Part model, mm, in its own coordinate system. A direction names the side the tool comes from. Give positions to 0.01 mm unless a question says otherwise; leave off trailing zeros. Write each loop counter-clockwise with the first axis right and the second up, starting at its lowest first coordinate (ties: lowest second). Pieces come first, ordered by that corner, then holes. Notation, with made-up numbers: M 3.25,52.25 L 21.25,52.25 A14 ccw 21.25,59.25 Z; hole C 58,84 d1. An arc over 180 degrees is marked long. Answer as CSV lines item,"result". Start each with the question number.
Item 1: Band-saw the part on C-C, the plane y = 0. Count the separate pieces of the cut face and the enclosed holes in it, then the cut area to 3 significant figures.
Item 2: Wall check: L1, parallel to Y at x = -40, z = 1.25 (3 decimals); L2, parallel to X at y = -12.5, z = 2; L3, parallel to Y at x = 14.5, z = 1.25. Give the ranges that are in metal, low to high. Write a range as from..to.
Item 3: Band-saw the part on B-B, the plane y = -10. List the corners of the cut face in (x, z).
Item 4: 3-axis set-ups, long thin cutter, end or side, ignore diameter. For faces 5 (the flat face through (0, 2.5, 19)), 6 (the cylindrical face through (-45.245, 25.361, 1.232)), 7 (the cylindrical face through (27.15, 26.99, 10.9)): which of +Z, -Z, +X, -X, +Y, -Y reach the whole face in a straight line?
Item 5: Two-plate mould, pull along X, no slides. Class faces 1 (the cylindrical face through (-25.361, -25.245, 9.895)), 2 (the cylindrical face through (46.99, -27.15, 1.73)), 3 (the cylindrical face through (-27.15, -26.99, 10.9)), 4 (the flat face through (34, 0, 5)): +X half, -X half, draft (parallel to the pull), parting line (faces both ways), or undercut.
Item 6: Pin check, flat tips, straight feed: pin 1 (10 mm diameter, centred on x = 40, y = 0, fed in from +Z); pin 2 (18.5 mm diameter, centred on x = 37, y = -9.5, fed in from +Z); pin 3 (3 mm diameter, centred on y = -10, z = 11.5, fed in from -X); pin 4 (10 mm diameter, centred on x = -38.5, y = -13.5, fed in from -Z). Stop position of each tip, or through.
Item 7: Band-saw the part on A-A, the plane z = 14.5. List the corners of the cut face in (x, y), then the cut area to 3 significant figures.
from build123d import *

# Parameters (mm, degrees)
F0_R     = 4.345
F1_DEPTH = 5
F3_DEPTH = 15
F4_T     = -2.5
F5_W     = 45
F5_H     = 5
F6_DEPTH = 20.001
F7_R     = 1.5


with BuildPart() as f1:
    # F0 (on Top) → F1 (new body)
    with BuildSketch(Plane.XY):
        with BuildLine():
            Line((40, 30), (-40, 30))
            ThreePointArc((-40, 30), (-47.0710678119, 27.0710678119), (-50, 20))
            Line((-50, 20), (-50, -20))
            ThreePointArc((-50, -20), (-47.0710678119, -27.0710678119), (-40, -30))
            Line((-40, -30), (40, -30))
            ThreePointArc((40, -30), (47.0710678119, -27.0710678119), (50, -20))
            Line((50, -20), (50, 20))
            ThreePointArc((50, 20), (47.0710678119, 27.0710678119), (40, 30))
        make_face()
        with Locations((-40, 0)):
            Circle(F0_R, mode=Mode.SUBTRACT)
        with Locations((40, 0)):
            Circle(F0_R, mode=Mode.SUBTRACT)
    extrude(amount=F1_DEPTH)

    # F2 (on face) → F3 (join)
    with BuildSketch(Plane.XY.offset(5)):
        with BuildLine():
            Line((20, 30), (-20, 30))
            ThreePointArc((-20, 30), (-27.0710678119, 27.0710678119), (-30, 20))
            Line((-30, 20), (-30, -20))
            ThreePointArc((-30, -20), (-27.0710678119, -27.0710678119), (-20, -30))
            Line((-20, -30), (20, -30))
            ThreePointArc((20, -30), (27.0710678119, -27.0710678119), (30, -20))
            Line((30, -20), (30, 20))
            ThreePointArc((30, 20), (27.0710678119, 27.0710678119), (20, 30))
        make_face()
    extrude(amount=F3_DEPTH)

    # F4
    f4_openings = [f1.faces().sort_by_distance(p)[0] for p in [
        (0, 0, 0),
    ]]
    offset(amount=F4_T, openings=f4_openings, kind=Kind.INTERSECTION)

    # F5 (on face) → F6 (cut, through all)
    with BuildSketch(Plane.XY.offset(20)):
        Rectangle(F5_W, F5_H)
    extrude(amount=-F6_DEPTH, mode=Mode.SUBTRACT)

    # F7
    f7_edges = [f1.edges().sort_by_distance(p)[0] for p in [
        (-22.5, 2.5, 18.75),
        (-22.5, -2.5, 18.75),
        (22.5, 2.5, 18.75),
        (22.5, -2.5, 18.75),
        (30, 0, 20),
        (27.071068, -27.071068, 20),
        (0, -30, 20),
        (47.071068, 27.071068, 5),
        (-30, -30, 5),
    ]]
    fillet(f7_edges, radius=F7_R)


solid = f1.part
Output:
1,separate pieces,"4"
1,enclosed holes,"0"
1,area,"205 mm²"
2,L1,"-30..-27.5, -6.845..-4.345, 4.345..6.845, 27.5..30"
2,L2,"-50..-47.5, 47.5..50"
2,L3,"-30..-27.5, 27.5..30"
3,outline,"M -50,0 L -47.5,0 L -47.5,2.5 L -27.5,2.5 L -27.5,17.5 L 27.5,17.5 L 27.5,2.5 L 47.5,2.5 L 47.5,0 L 50,0 L 50,3.5 A1.5 ccw 48.5,5 L 30,5 L 30,18.5 A1.5 ccw 28.5,20 L -28.5,20 A1.5 ccw -30,18.5 L -30,5 L -48.5,5 A1.5 ccw -50,3.5 Z"
4,face 5,"+Z, -Z"
4,face 6,"-Z"
4,face 7,"+Z, +X, +Y"
5,face 1,"undercut"
5,face 2,"+X half"
5,face 3,"-X half"
5,face 4,"draft"
6,pin 1,"z = 5"
6,pin 2,"z = 20"
6,pin 3,"x = -30"
6,pin 4,"z = 2.5"
7,outline,"M -30,-20 A10 ccw -20,-30 L 20,-30 A10 ccw 30,-20 L 30,20 A10 ccw 20,30 L -20,30 A10 ccw -30,20 Z; hole M -27.5,-20 A7.5 ccw -20,-27.5 L 20,-27.5 A7.5 ccw 27.5,-20 L 27.5,20 A7.5 ccw 20,27.5 L -20,27.5 A7.5 ccw -27.5,20 Z"
7,area,"537 mm²"
